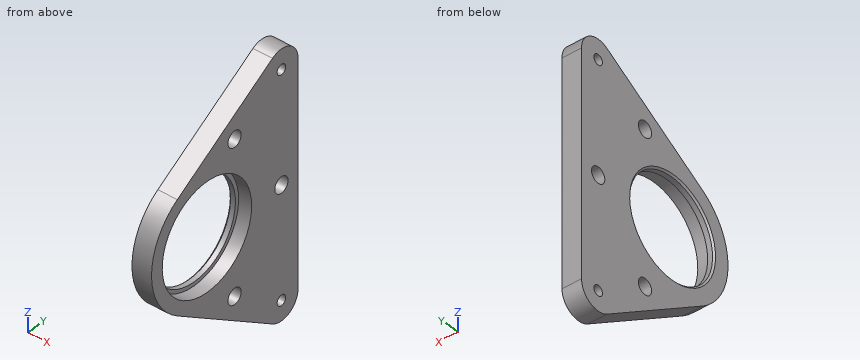
from build123d import *

# Parameters (mm, degrees)
SKETCH1_R           = 20
SKETCH1_R_2         = 15
BOSS_EXTRUDE1_DEPTH = 2
SKETCH2_R           = 20
SKETCH2_R_2         = 16
BOSS_EXTRUDE2_DEPTH = 4
SKETCH3_R           = 2
BOSS_EXTRUDE3_DEPTH = 6
SKETCH4_R           = 2.4
CUT_EXTRUDE1_DEPTH  = 6
SKETCH5_R           = 2
SKETCH5_R_2         = 1.55
BOSS_EXTRUDE4_DEPTH = 6
SKETCH6_R           = 16.15
SKETCH6_R_2         = 16
CUT_EXTRUDE2_DEPTH  = 4
CHAMFER1_SIZE       = 0.5


with BuildPart() as part:
    # Sketch1 → Boss-Extrude1 (new body)
    with BuildSketch(Plane(origin=(0, 0, 0), x_dir=(0, 0, -1), z_dir=(1, 0, 0))):
        Circle(SKETCH1_R)
        Circle(SKETCH1_R_2, mode=Mode.SUBTRACT)
    extrude(amount=BOSS_EXTRUDE1_DEPTH)

    # Sketch2 → Boss-Extrude2 (add)
    with BuildSketch(Plane(origin=(2, 0, 0), x_dir=(0, 0, -1), z_dir=(1, 0, 0))):
        Circle(SKETCH2_R)
        Circle(SKETCH2_R_2, mode=Mode.SUBTRACT)
    extrude(amount=BOSS_EXTRUDE2_DEPTH)

    # Sketch3 → Boss-Extrude3 (add)
    with BuildSketch(Plane(origin=(6, 0, 0), x_dir=(0, 0, -1), z_dir=(1, 0, 0))):
        with BuildLine():
            Line((-38.608830959, 23.677807584), (-16.909895057, -10.679674581))
            ThreePointArc((-16.909895057, -10.679674581), (0, 20), (16.909895057, -10.679674581))
            Line((16.909895057, -10.679674581), (38.608830959, 23.677807584))
            ThreePointArc((38.608830959, 23.677807584), (38.790546744, 29.777964933), (33.535862442, 32.881709959))
            Line((33.535862442, 32.881709959), (-33.535862442, 32.881709959))
            ThreePointArc((-33.535862442, 32.881709959), (-38.790546744, 29.777964933), (-38.608830959, 23.677807584))
        make_face()
        with Locations((-33.535862442, 26.881709959)):
            Circle(SKETCH3_R, mode=Mode.SUBTRACT)
        with Locations((33.535862442, 26.881709959)):
            Circle(SKETCH3_R, mode=Mode.SUBTRACT)
    extrude(amount=-BOSS_EXTRUDE3_DEPTH)

    # Sketch4 → Cut-Extrude1 (cut)
    with BuildSketch(Plane(origin=(6, 0, 0), x_dir=(0, 0, -1), z_dir=(1, 0, 0))):
        with Locations((-22.856187861, 9.971814902)):
            Circle(SKETCH4_R)
        with Locations((22.856187861, 9.971814902)):
            Circle(SKETCH4_R)
        with Locations((0, 26.881709959)):
            Circle(SKETCH4_R)
    extrude(amount=-CUT_EXTRUDE1_DEPTH, mode=Mode.SUBTRACT)

    # Sketch5 → Boss-Extrude4 (add)
    with BuildSketch(Plane(origin=(0, 0, 0), x_dir=(0, 0, -1), z_dir=(1, 0, 0))):
        with Locations((33.535862442, 26.881709959)):
            Circle(SKETCH5_R)
        with Locations((33.535862442, 26.881709959)):
            Circle(SKETCH5_R_2, mode=Mode.SUBTRACT)
        with Locations((-33.535862442, 26.881709959)):
            Circle(SKETCH5_R)
        with Locations((-33.535862442, 26.881709959)):
            Circle(SKETCH5_R_2, mode=Mode.SUBTRACT)
    extrude(amount=BOSS_EXTRUDE4_DEPTH)

    # Sketch6 → Cut-Extrude2 (cut)
    with BuildSketch(Plane(origin=(6, 0, 0), x_dir=(0, 0, -1), z_dir=(1, 0, 0))):
        Circle(SKETCH6_R)
        Circle(SKETCH6_R_2, mode=Mode.SUBTRACT)
    extrude(amount=-CUT_EXTRUDE2_DEPTH, mode=Mode.SUBTRACT)

    # Chamfer1
    chamfer1_edges = [part.edges().sort_by_distance(p)[0] for p in [
        (0, 0, 15),
    ]]
    chamfer(chamfer1_edges, length=CHAMFER1_SIZE)


solid = part.part
Geometry check sheet. Reference: the model listing, model coordinates, mm. Round coordinates to 2 decimals unless told otherwise and drop trailing zeros. Loops run counter-clockwise (first coordinate to the right, second up) from the corner with the lowest first, then second, coordinate; pieces in that order, holes last.
Item 1: Cross-section at C-C on y = 0. Record the boundary of the cut face in (x, z).
Item 2: Cross-section at A-A on z = 0. Record the boundary of the cut face in (x, y).
Item 3: Cross-section at B-B on x = 4. Record the boundary of the cut face in (y, z), then the cut area to 3 significant figures.
Item 4: Gauge pin test, flat ends, axial feed: pin 1 (18 mm diameter, centred on y = 0, z = 0, fed in from -X); pin 2 (1.5 mm diameter, centred on x = 4.5, y = 23, fed in from -Z). Record the tip position at first contact, or that the pin passes through.
Item 5: Thickness scan on line 1 (Y direction, x = 3.6, z = 0); line 2 (Y direction, x = 0.9, z = 0); line 3 (Z direction, x = 5.3, y = -3). Record the ranges inside material, lowest first.
Item 6: Cross-section at D-D on z = 18. Record the boundary of the cut face in (x, y).
Answer sheet:
1. outline: (0, -23.65) - (6, -23.65) - (6, -16.15) - (2, -16.15) - (2, -15) - (0.5, -15) - (0, -15.5) - close; (0, 15.5) - (0.5, 15) - (2, 15) - (2, 16.15) - (6, 16.15) - (6, 23.65) - (0, 23.65) - close
2. outline: (0, -20) - (6, -20) - (6, -16.15) - (2, -16.15) - (2, -15) - (0.5, -15) - (0, -15.5) - close; (0, 15.5) - (0.5, 15) - (2, 15) - (2, 16.15) - (6, 16.15) - (6, 24.48) - (0, 24.48) - close; (0, 29.28) - (6, 29.28) - (6, 32.88) - (0, 32.88) - close
3. outline: (-10.68, -16.91) - (23.68, -38.61) arc R6 ccw to (32.88, -33.54) - (32.88, 33.54) arc R6 ccw to (23.68, 38.61) - (-10.68, 16.91) arc R20 ccw to start; hole circle Ø32.3 at (0, 0); hole circle Ø4.8 at (9.97, -22.86); hole circle Ø4.8 at (9.97, 22.86); hole circle Ø4.8 at (26.88, 0); hole circle Ø3.1 at (26.88, -33.54); hole circle Ø3.1 at (26.88, 33.54)
3. area: 1,950 mm2
4. pin 1: passes through
4. pin 2: stops at z = -38.65
5. line 1: y = -20 to -16.15, 16.15 to 24.48, 29.28 to 32.88
5. line 2: y = -20 to -15, 15 to 24.48, 29.28 to 32.88
5. line 3: z = -21.76 to -15.87, 15.87 to 21.76
6. outline: (0, -8.95) - (6, -8.95) - (6, 32.88) - (0, 32.88) - close
